For this review, take the finished solid that the model builds, in its own axes (mm). A direction names the side the tool comes from. Coordinates: 2 decimals unless noted, no trailing zeros. Loops run counter-clockwise (first coordinate to the right, second up) from the corner with the lowest first, then second, coordinate; pieces in that order, holes last. Notation, with made-up numbers: (70, -11) - (78, -11) arc R13 cw to (78, 1) - close; hole circle Ø8 at (31, -19). An arc over 180 degrees is marked (long way). Use one line per item in the form item = value. Start each with the question number.
1. Machinability: for faces 1 (the face through (-25, 146, 7.5)), 2 (the face through (-5.4, 160, -0.3)), 3 (the face through (-27.5, 84, 0)), which of the approach directions +Z, -Z, +X, -X, +Y, -Y give a long, thin tool a straight path to every point of the face, cutting with its end or side? Answer none if there is none.
2. Add section A-A on x = 0. Give the boundary of the cut face in (y, z).
3. For pin 1 Ø5 at (x, z) = (-7, -14.5) entering from -Y, flat-tipped, find the tip position at first contact; note if it passes through.
4. To check wall thickness, follow probe 1 along X at (y, z) = (141, -13.5); probe 2 along X at (y, z) = (166, 0). State the ranges of each line that lie inside material, in increasing order.
5. Draft analysis for pull direction Y (two halves, no side actions). For faces 4 (the face through (0, 170, -6)), 5 (the face through (0, 84, -27.5)), 6 (the face through (-25, 146, -7.5)), state which applies: +Y half, -Y half, draft (parallel to the pull), parting line (faces both ways), or undercut.
6. Add section B-B on z = 0. Give the boundary of the cut face in (x, y).
7. Add section C-C on y = 10. Give the boundary of the cut face in (x, z) (3 decimals).
8. Add section D-D on y = 60. Give the boundary of the cut face in (x, z), and give its area (3 significant figures).
```python
from build123d import *

# Parameters (mm, degrees)
SKETCH1_W                         = 55
SKETCH1_H                         = 55
BOSS_EXTRUDE1_DEPTH               = 170
SKETCH2_W                         = 46
SKETCH2_H                         = 46
CUT_EXTRUDE4_DEPTH                = 160
SKETCH5_W                         = 14.999999972
SKETCH5_H                         = 5
CUT_EXTRUDE5_DEPTH                = 4.5
TAP_DRILL_FOR_M4_TAP1_D           = 3.3
TAP_DRILL_FOR_M4_TAP1_CSINK_D     = 3.35
TAP_DRILL_FOR_M4_TAP1_CSINK_ANGLE = 90
SKETCH8_R                         = 5
CUT_EXTRUDE6_DEPTH                = 175.391800266


with BuildPart() as part:
    # Sketch1 → Boss-Extrude1 (new body)
    with BuildSketch(Plane(origin=(0, 0, 0), x_dir=(1, 0, 0), z_dir=(0, 1, 0))):
        Rectangle(SKETCH1_W, SKETCH1_H)
    extrude(amount=BOSS_EXTRUDE1_DEPTH)

    # Sketch2 → Cut-Extrude4 (cut)
    with BuildSketch(Plane(origin=(0, 0, 0), x_dir=(1, 0, 0), z_dir=(0, 1, 0))):
        Rectangle(SKETCH2_W, SKETCH2_H)
    extrude(amount=CUT_EXTRUDE4_DEPTH, mode=Mode.SUBTRACT)

    # Sketch5 → Cut-Extrude5 (cut)
    with BuildSketch(Plane.ZY.offset(27.5)):
        with Locations((1.4e-08, 145.67539027)):
            Rectangle(SKETCH5_W, SKETCH5_H)
    extrude(amount=-CUT_EXTRUDE5_DEPTH, mode=Mode.SUBTRACT)

    # Tap Drill for M4 Tap1 (through all)
    with Locations(Plane(origin=(13.784, 10.000000066, -27.5), x_dir=(-1, 0, 0), z_dir=(0, 0, -1))):
        with Locations((0, 0), (27.5, 0)):
            CounterSinkHole(TAP_DRILL_FOR_M4_TAP1_D / 2, TAP_DRILL_FOR_M4_TAP1_CSINK_D / 2, counter_sink_angle=TAP_DRILL_FOR_M4_TAP1_CSINK_ANGLE)

    # Sketch8 → Cut-Extrude6 (cut, through all)
    with BuildSketch(Plane(origin=(0, 170, 0), x_dir=(1, 0, 0), z_dir=(0, 1, 0))):
        with Locations(Location((0, 0, 0), (0, 0, 270))):
            Circle(SKETCH8_R)
    extrude(amount=-CUT_EXTRUDE6_DEPTH, mode=Mode.SUBTRACT)


solid = part.part
```
Conclusion:
q1.face_1 = -X
q1.face_2 = -Y
q1.face_3 = +Z, -Z, -X, +Y, -Y
q2.outline = (0, -27.5) - (170, -27.5) - (170, -5) - (160, -5) - (160, -23) - (0, -23) - close; (0, 23) - (160, 23) - (160, 5) - (170, 5) - (170, 27.5) - (0, 27.5) - close
q3.pin_1 = 160
q4.probe_1 = -27.5 to -23, 23 to 27.5
q4.probe_2 = -27.5 to -5, 5 to 27.5
q5.face_4 = +Y half
q5.face_5 = draft
q5.face_6 = undercut
q6.outline = (-27.5, 0) - (-23, 0) - (-23, 143.18) - (-27.5, 143.18) - close; (-27.5, 148.18) - (-23, 148.18) - (-23, 160) - (-5, 160) - (-5, 170) - (-27.5, 170) - close; (5, 160) - (23, 160) - (23, 0) - (27.5, 0) - (27.5, 170) - (5, 170) - close
q7.outline = (-27.5, -27.5) - (-15.391, -27.5) - (-15.366, -27.475) - (-15.366, -23) - (-23, -23) - (-23, 23) - (-15.366, 23) - (-15.366, 27.5) - (-27.5, 27.5) - close; (-12.066, -27.475) - (-12.041, -27.5) - (12.109, -27.5) - (12.134, -27.475) - (12.134, -23) - (-12.066, -23) - close; (-12.066, 23) - (12.134, 23) - (12.134, 27.5) - (-12.066, 27.5) - close; (15.434, -27.475) - (15.459, -27.5) - (27.5, -27.5) - (27.5, 27.5) - (15.434, 27.5) - (15.434, 23) - (23, 23) - (23, -23) - (15.434, -23) - close
q8.outline = (-27.5, -27.5) - (27.5, -27.5) - (27.5, 27.5) - (-27.5, 27.5) - close; hole (-23, -23) - (23, -23) - (23, 23) - (-23, 23) - close
q8.area = 909 mm^2
